```python
from build123d import *

# Parameters (mm, degrees)
F0_W     = 16
F0_H     = 16
F1_DEPTH = 10
F2_T     = -1.5
F3_R     = 2.425
F4_DEPTH = 1.7
F5_R     = 2.925
F6_DEPTH = 10


with BuildPart() as f1:
    # F0 (on Top) → F1 (new body)
    with BuildSketch(Plane.XY):
        Rectangle(F0_W, F0_H)
    extrude(amount=F1_DEPTH)

    # F2
    f2_openings = [f1.faces().sort_by_distance(p)[0] for p in [
        (0, 0, 0),
    ]]
    offset(amount=F2_T, openings=f2_openings)

    # F3 (on face) → F4 (join)
    with BuildSketch(Plane.XY.offset(10)):
        with Locations((-4, -4)):
            Circle(F3_R)
        with Locations((-4, 4)):
            Circle(F3_R)
        with Locations((4, -4)):
            Circle(F3_R)
        with Locations((4, 4)):
            Circle(F3_R)
    extrude(amount=F4_DEPTH)

    # F5 (on Top) → F6 (join)
    with BuildSketch(Plane.XY):
        Circle(F5_R)
    extrude(amount=F6_DEPTH)


solid = f1.part
```
The model under review builds one solid part; all positions refer to its coordinate system, in mm. A direction names the side the tool comes from. Round coordinates to 2 decimals unless told otherwise and drop trailing zeros. Write each loop counter-clockwise with the first axis right and the second up, starting at its lowest first coordinate (ties: lowest second). Pieces come first, ordered by that corner, then holes.
(1) Wall thickness on L1, parallel to X at y = 1, z = 7; L2, parallel to Y at x = 0.5, z = 1; L3, parallel to Y at x = 0.75, z = 4.5: over which ranges is each line inside the solid? List them lowest first.
(2) We need section D-D on x = -7. Give the boundary of the cut face in (y, z).
(3) Insertion check: pin 1 (5 mm diameter, centred on x = -3.5, y = 0, fed in from +Z). The pin has a flat end and moves straight along its axis. Give the tip position at first contact, or say it passes through.
(4) We need section A-A on x = -4. Give the boundary of the cut face in (y, z) (3 decimals), and give its area (3 significant figures).
(5) We need section C-C on z = 10.5. Give the boundary of the cut face in (x, y) (3 decimals), and give its area (3 significant figures).
(6) Mouldability with a two-part tool opening along Y and no side actions: class faces 4 (the flat face through (-8, 0, 5)), 5 (the flat face through (0, 8, 5)), 6 (the flat face through (-6.5, 0, 4)) as +Y half, -Y half, draft (parallel to the pull), parting line (faces both ways), or undercut.
(7) Machinability: for faces 1 (the cylindrical face through (6.313, -3.272, 10.838)), 2 (the flat face through (0, 6.5, 4)), 3 (the flat face through (7, 0, 0)), which of the approach directions +Z, -Z, +X, -X, +Y, -Y give a long, thin tool a straight path to every point of the face, cutting with its end or side? Answer none if there is none.
Findings below:
1. L1: x = -8 to -6.5, -2.75 to 2.75, 6.5 to 8
1. L2: y = -8 to -6.5, -2.88 to 2.88, 6.5 to 8
1. L3: y = -8 to -6.5, -2.83 to 2.83, 6.5 to 8
2. outline: (-8, 0) - (8, 0) - (8, 10) - (-8, 10) - close
3. pin 1: stops at z = 11.7
4. outline: (-8, 0) - (-6.5, 0) - (-6.5, 8.5) - (6.5, 8.5) - (6.5, 0) - (8, 0) - (8, 10) - (6.425, 10) - (6.425, 11.7) - (1.575, 11.7) - (1.575, 10) - (-1.575, 10) - (-1.575, 11.7) - (-6.425, 11.7) - (-6.425, 10) - (-8, 10) - close
4. area: 66.0 mm2
5. outline: circle Ø4.85 at (-4, -4); circle Ø4.85 at (-4, 4); circle Ø4.85 at (4, -4); circle Ø4.85 at (4, 4)
5. area: 73.9 mm2
6. face 4: draft
6. face 5: +Y half
6. face 6: undercut
7. face 1: +Z
7. face 2: -Z
7. face 3: -Z, +X, -X, +Y, -Y
